Can you work these out from the model? Positions are in its coordinate system, mm. A direction names the side the tool comes from. Give positions to 0.01 mm unless a question says otherwise; leave off trailing zeros. Order: outer loops, then holes, each group sorted by start corner. A loop starts at its lowest first (then second) coordinate and runs counter-clockwise, first axis right, second up.
Item 1: Which directions (+Z, -Z, +X, -X, +Y, -Y) give clear straight access to the entire face, cutting with the end or side of a thin tool? Please do faces 4 (the flat face through (-6, 6.2, 8)), 5 (the flat face through (-4.75, 7, 8)), 6 (the flat face through (-12.75, 4, 3)).
Item 2: I want a section at A-A, the plane z = 0. Write out the boundary of the cut face in (x, y) (3 decimals), then the cut area to 3 significant figures.
Item 3: I'm going to push flat-ended pins straight in: pin 1 Ø4 at (x, y) = (1, 5.5) entering from +Z; pin 2 Ø2.5 at (x, z) = (5.5, 7) entering from -Y; pin 3 Ø3 at (x, z) = (-8, 0) entering from -Y. Where does each tip first touch, or does it pass through?
Item 4: If we mould it in two halves opening along X, with no side actions, what happens to faces 1 (the cylindrical face through (6.24, 4.04, 0.23)), 2 (the flat face through (12.75, 4, 4)), 3 (the flat face through (-10, 4, 12.2))? For each: +X half, -X half, draft (parallel to the pull), parting line (faces both ways), or undercut.
Item 5: I want a section at C-C, the plane z = 9. Write out the boundary of the cut face in (x, y).
Item 6: I want a section at D-D, the plane y = 4.75. Write out the boundary of the cut face in (x, z) (3 decimals), then the cut area to 3 significant figures.
Item 7: I want a section at B-B, the plane y = 7.25. Write out the boundary of the cut face in (x, z) (3 decimals), then the cut area to 3 significant figures.
Item 8: If I drill on line 1 along X through (y, z) = (4.25, 0) (3 decimals); line 2 along X through (y, z) = (7, 5.75); line 3 along X through (y, z) = (4.5, 8.75), over which ranges is the centre line in solid material (lowest first)?
```python
from build123d import *

# Parameters (mm, degrees)
SKETCH1_R           = 1.775
BOSS_EXTRUDE1_DEPTH = 6.2
BOSS_EXTRUDE2_START = 6.2
SKETCH1_3_R         = 1.775
BOSS_EXTRUDE2_DEPTH = 2


with BuildPart() as part:
    # Sketch1 → Boss-Extrude1 (new body)
    with BuildSketch(Plane(origin=(0, 0, 0), x_dir=(1, 0, 0), z_dir=(0, 1, 0))):
        Polygon((-12.75, 5), (12.75, 5), (12.75, -12.2), (7.75, -12.2), (7.75, -3.2), (-7.75, -3.2), (-7.75, -12.2), (-12.75, -12.2), align=None)
        with Locations(Location((-8, 0, 0), (0, 0, 90))):
            Circle(SKETCH1_R, mode=Mode.SUBTRACT)
        with Locations(Location((8, 0, 0), (0, 0, 90))):
            Circle(SKETCH1_R, mode=Mode.SUBTRACT)
    extrude(amount=BOSS_EXTRUDE1_DEPTH)

    # Sketch1<3> → Boss-Extrude2 (add)
    with BuildSketch(Plane(origin=(0, 0, 0), x_dir=(1, 0, 0), z_dir=(0, 1, 0)).offset(BOSS_EXTRUDE2_START)):
        Polygon((12.75, 5), (-12.75, 5), (-12.75, -12.2), (-4.75, -12.2), (-4.75, -3.2), (4.75, -3.2), (4.75, -12.2), (12.75, -12.2), align=None)
        with Locations(Location((-8, 0, 0), (0, 0, 90))):
            Circle(SKETCH1_3_R, mode=Mode.SUBTRACT)
        with Locations(Location((8, 0, 0), (0, 0, 90))):
            Circle(SKETCH1_3_R, mode=Mode.SUBTRACT)
    extrude(amount=BOSS_EXTRUDE2_DEPTH)


solid = part.part
```
Results list:
1. face 4: +Z, -Y
1. face 5: +Z, +Y, -Y
1. face 6: +Z, -Z, -X, +Y, -Y
2. outline: (-12.75, 0) - (-9.775, 0) - (-9.775, 8.2) - (-12.75, 8.2) - close; (-6.225, 0) - (6.225, 0) - (6.225, 8.2) - (-6.225, 8.2) - close; (9.775, 0) - (12.75, 0) - (12.75, 8.2) - (9.775, 8.2) - close
2. area: 151 mm2
3. pin 1: stops at z = 3.2
3. pin 2: stops at y = 6.2
3. pin 3: passes through
4. face 1: undercut
4. face 2: +X half
4. face 3: draft
5. outline: (-12.75, 0) - (-7.75, 0) - (-7.75, 6.2) - (-4.75, 6.2) - (-4.75, 8.2) - (-12.75, 8.2) - close; (4.75, 6.2) - (7.75, 6.2) - (7.75, 0) - (12.75, 0) - (12.75, 8.2) - (4.75, 8.2) - close
6. outline: (-12.75, -5) - (12.75, -5) - (12.75, 12.2) - (7.75, 12.2) - (7.75, 3.2) - (-7.75, 3.2) - (-7.75, 12.2) - (-12.75, 12.2) - close; hole circle Ø3.55 at (-8, 0); hole circle Ø3.55 at (8, 0)
6. area: 279 mm2
7. outline: (-12.75, -5) - (12.75, -5) - (12.75, 12.2) - (4.75, 12.2) - (4.75, 3.2) - (-4.75, 3.2) - (-4.75, 12.2) - (-12.75, 12.2) - close; hole circle Ø3.55 at (-8, 0); hole circle Ø3.55 at (8, 0)
7. area: 333 mm2
8. line 1: x = -12.75 to -9.775, -6.225 to 6.225, 9.775 to 12.75
8. line 2: x = -12.75 to -4.75, 4.75 to 12.75
8. line 3: x = -12.75 to -7.75, 7.75 to 12.75
